Autodesk Inventor part; units mm, degrees
ref_plane "Work Plane1" through (0, 0, 203.2) normal (0, 0, 1) x (1, 0, 0)
ref_plane "Work Plane2" through (0, 0, 200.025) normal (0, 0, 1) x (1, 0, 0)
ref_plane "YZ Plane" through (0, 0, 0) normal (1, 0, 0) x (0, 1, 0)
sketch "Sketch1" plane through (0, 0, 0) normal (0, 0, 1) x (1, 0, 0)
  line L0 (-251.1425, 0) -> (251.1425, 0) construction
  line L1 (0, -146.685) -> (0, 146.685) construction
  line L2 (-179.3875, 104.775) -> (179.3875, 104.775)
  line L3 (179.3875, 104.775) -> (179.3875, -104.775)
  line L4 (179.3875, -104.775) -> (-179.3875, -104.775)
  line L5 (-179.3875, -104.775) -> (-179.3875, 104.775)
  point P0 (0, 0)
  point P1 (0, 104.775)
  point P2 (-179.3875, 0)
  dimension "d0" = 358.775
  dimension "d1" = 209.55
ref_plane "Work Plane1" through (0, 0, 203.2) normal (0, 0, 1) x (1, 0, 0)
sketch "Sketch2" plane through (0, 0, 203.2) normal (0, 0, 1) x (1, 0, 0)
  line L0 (0, -146.685) -> (0, 146.685) construction
  line L1 (-253.365, 0) -> (253.365, 0) construction
  line L2 (-128.5875, 53.975) -> (128.5875, 53.975)
  line L3 (128.5875, 53.975) -> (128.5875, -53.975)
  line L4 (128.5875, -53.975) -> (-128.5875, -53.975)
  line L5 (-128.5875, -53.975) -> (-128.5875, 53.975)
  line L6 (-179.3875, 104.775) -> (179.3875, 104.775) construction
  line L7 (-179.3875, -104.775) -> (-179.3875, 104.775) construction
  point P0 (0, 0)
  point P1 (0, 53.975)
  point P2 (-128.5875, 0)
  dimension "d3" = 50.8
  dimension "d4" = 50.8
loft "Loft1" add profiles "Sketch1", "Sketch2"
sketch "Sketch3" plane through (179.3875, 104.775, 0) normal (0, 0, -1) x (-1, 0, 0)
  line L0 (179.3875, -251.46) -> (179.3875, 41.91) construction
  line L1 (430.53, -104.775) -> (-71.755, -104.775) construction
  line L2 (3.175, -3.175) -> (28.575, -3.175) construction
  line L3 (355.6, -3.175) -> (355.6, -28.575) construction
  line L4 (355.6, -206.375) -> (330.2, -206.375) construction
  line L5 (3.175, -206.375) -> (3.175, -180.975) construction
  line L6 (28.575, -3.175) -> (28.575, -28.575)
  line L7 (28.575, -28.575) -> (3.175, -28.575)
  line L8 (3.175, -180.975) -> (28.575, -180.975)
  line L9 (28.575, -180.975) -> (28.575, -206.375)
  line L10 (330.2, -3.175) -> (330.2, -28.575)
  line L11 (330.2, -28.575) -> (355.6, -28.575)
  line L12 (330.2, -206.375) -> (330.2, -180.975)
  line L13 (330.2, -180.975) -> (355.6, -180.975)
  line L14 (3.175, -28.575) -> (3.175, -3.175) construction
  line L15 (28.575, -3.175) -> (330.2, -3.175)
  line L16 (330.2, -3.175) -> (355.6, -3.175) construction
  line L17 (355.6, -28.575) -> (355.6, -180.975)
  line L18 (355.6, -180.975) -> (355.6, -206.375) construction
  line L19 (330.2, -206.375) -> (28.575, -206.375)
  line L20 (28.575, -206.375) -> (3.175, -206.375) construction
  line L21 (3.175, -180.975) -> (3.175, -28.575)
  line L22 (0, 0) -> (0, -209.55) construction
  line L23 (358.775, 0) -> (0, 0) construction
  point P0 (179.3875, -104.775)
  point P1 (179.3875, -3.175)
  point P2 (3.175, -104.775)
  dimension "d9" = 3.175
  dimension "d10" = 3.175
  dimension "d11" = 25.4
ref_plane "Work Plane2" through (0, 0, 200.025) normal (0, 0, 1) x (1, 0, 0)
sketch "Sketch5" plane through (0, 0, 200.025) normal (0, 0, 1) x (1, 0, 0)
  line L0 (150.8125, 101.6) -> (150.8125, 76.2)
  line L1 (150.8125, 76.2) -> (176.2125, 76.2)
  line L2 (176.2125, -76.2) -> (176.2125, 76.2)
  line L3 (176.2125, -76.2) -> (150.8125, -76.2)
  line L4 (150.8125, -76.2) -> (150.8125, -101.6)
  line L5 (-150.8125, -101.6) -> (150.8125, -101.6)
  line L6 (-150.8125, -101.6) -> (-150.8125, -76.2)
  line L7 (-150.8125, -76.2) -> (-176.2125, -76.2)
  line L8 (-176.2125, 76.2) -> (-176.2125, -76.2)
  line L9 (-150.8125, 76.2) -> (-176.2125, 76.2)
  line L10 (-150.8125, 101.6) -> (-150.8125, 76.2)
  line L11 (150.8125, 101.6) -> (-150.8125, 101.6)
  line L12 (-100.0125, 50.8) -> (-100.0125, 25.4)
  line L13 (-100.0125, 25.4) -> (-125.4125, 25.4)
  line L14 (-125.4125, 25.4) -> (-125.4125, -25.4)
  line L15 (-125.4125, -25.4) -> (-100.0125, -25.4)
  line L16 (-100.0125, -25.4) -> (-100.0125, -50.8)
  line L17 (-100.0125, -50.8) -> (100.0125, -50.8)
  line L18 (100.0125, -50.8) -> (100.0125, -25.4)
  line L19 (100.0125, -25.4) -> (125.4125, -25.4)
  line L20 (125.4125, -25.4) -> (125.4125, 25.4)
  line L21 (125.4125, 25.4) -> (100.0125, 25.4)
  line L22 (100.0125, 25.4) -> (100.0125, 50.8)
  line L23 (100.0125, 50.8) -> (-100.0125, 50.8)
  line L24 (-128.5875, 53.975) -> (128.5875, 53.975)
  point P0 (0, 0)
  dimension "d15" = 3.175
loft "Loft2" cut profiles "Sketch3", "Sketch5" contours all / L23 L22 L21 L20 L19 L18 L17 L16 L15 L14 L13 L12
sketch "Sketch6" plane through (179.3875, 104.775, 0) normal (0, 0, -1) x (-1, 0, 0)
  line L0 (430.53, -104.775) -> (-71.755, -104.775) construction
  line L1 (179.3875, -251.46) -> (179.3875, 41.91) construction
  line L2 (15.875, -15.875) -> (342.9, -15.875) construction
  line L3 (342.9, -15.875) -> (342.9, -193.675) construction
  line L4 (342.9, -193.675) -> (15.875, -193.675) construction
  line L5 (15.875, -193.675) -> (15.875, -15.875) construction
  line L6 (3.175, -28.575) -> (28.575, -28.575) construction
  line L7 (28.575, -28.575) -> (28.575, -3.175) construction
  circle A0 centre (15.875, -15.875) radius 3.175
  circle A1 centre (342.9, -15.875) radius 3.175
  circle A2 centre (342.9, -193.675) radius 3.175
  circle A3 centre (15.875, -193.675) radius 3.175
  point P0 (179.3875, -104.775)
  point P1 (179.3875, -15.875)
  point P2 (15.875, -104.775)
  dimension "d20" = 12.7
  dimension "d21" = 12.7
  dimension "d22" = 6.35
extrude "Extrusion1" cut sketch "Sketch6" against normal through all
equation "\"d21\" = d20"
properties part number "Front Cover"
CAD build for the part. Positions are in the model's coordinates, mm. Round coordinates to 2 decimals unless told otherwise and drop trailing zeros. Return JSON: item names as keys, results as strings. Group by question number.
(1) Drop flat-ended pins along their axis: P1, Ø3, axis at x = -143, z = 117.5, coming from the +Y side (3 decimals); P2, Ø6, axis at x = 15, z = 54.5, coming from the +Y side; P3, Ø3, axis at y = -81.5, z = 35.5, coming from the +X side. Give the stop position or say it passes through.
(2) Wall check: probe 1 along Z at (x, y) = (-47, 47) (3 decimals); probe 2 along X at (y, z) = (-88, 37); probe 3 along X at (y, z) = (88.9, 34). Give the ranges that are in metal, low to high. Write a range as [from, to].
(3) Saw through at A-A, the plane z = 39. Give the number of separate pieces and of enclosed holes in the cut face, and give its area (3 significant figures).
(4) Mould opens along Y. For faces 1 (the flat face through (-1, 2, 203.2)), 2 (the flat face through (2, 0, 200.025)) say: +Y half, -Y half, draft (parallel to the pull), parting line (faces both ways), or undercut.
Answer list:
{
 "1": {"P1": "y = 75.775", "P2": "y = 91.9", "P3": "x = 170.89"},
 "2": {"probe 1": "[200.025, 203.2]", "probe 2": "[-170.14, -166.56], [-160.47, -141.42], [141.42, 160.47], [166.56, 170.14]", "probe 3": "[-170.89, -166.69], [-160.34, -142.18], [142.18, 160.34], [166.69, 170.89]"},
 "3": {"separate pieces": "1", "enclosed holes": "5", "area": "5,930 mm2"},
 "4": {"face 1": "draft", "face 2": "undercut"}
}
